Could you check a few things on this drawing? It's one solid part, dimensions in mm from its lowest x, y, z. A direction names the side the tool comes from. Give positions to 0.01 mm unless a question says otherwise; leave off trailing zeros. Write each loop counter-clockwise with the first axis right and the second up, starting at its lowest first coordinate (ties: lowest second). Pieces come first, ordered by that corner, then holes. Notation, with made-up numbers: M 88.25,24.5 L 109.25,24.5 A17 ccw 109.25,44.5 Z; hole C 32.25,16 d2. An arc over 180 degrees is marked long. Write each question's results on one line, items separated by ' | '.
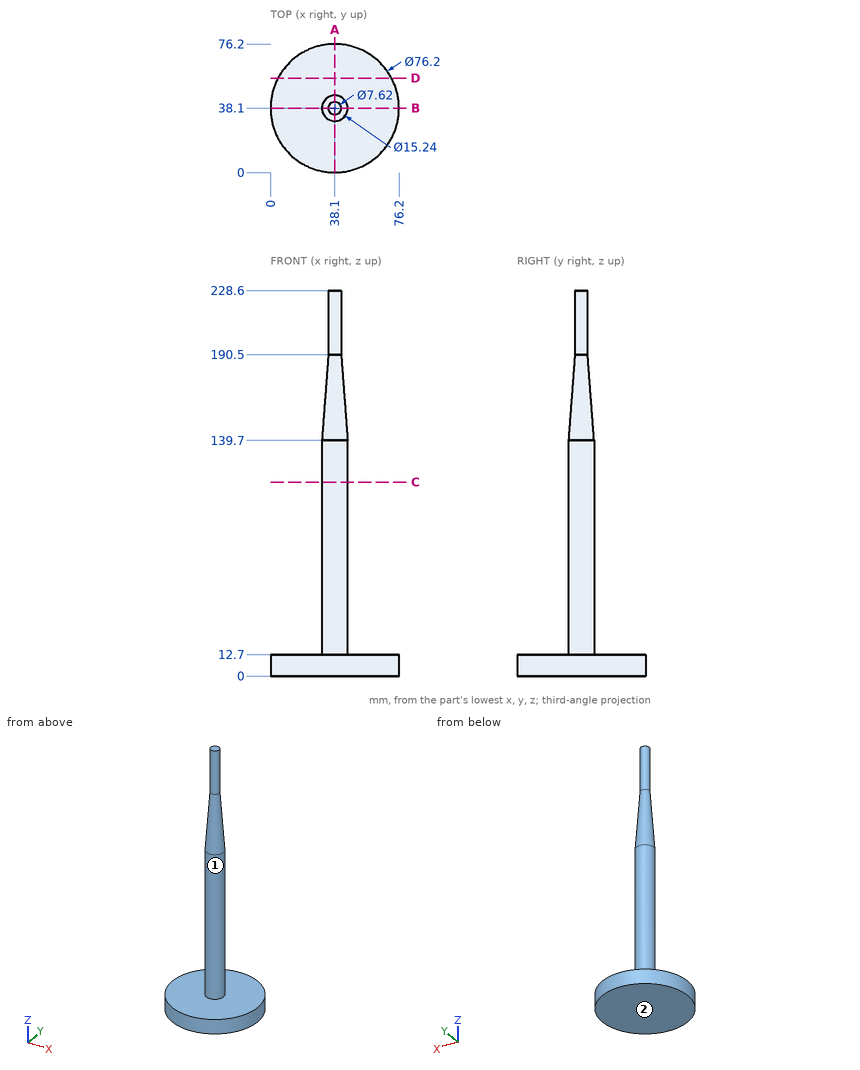
Item 1: For the marked faces 1 and 2, which set-ups out of +Z, -Z, +X, -X, +Y, -Y let a thin tool reach every point of the face, with its end or its side?
Geometry says:
face 1: +Z | face 2: -Z, +X, -X, +Y, -Y
Item 2: I want a section at D-D, the plane y = 56. Please give me the cut outline in (x, z).
Geometry says:
outline: M 4.47,0 L 71.73,0 L 71.73,12.7 L 4.47,12.7 Z
Item 3: I'm going to push flat-ended pins straight in: pin 1 (4 mm diameter, centred on x = 29.5, z = 75, fed in from +Y); pin 2 (10 mm diameter, centred on y = 35, z = 177.5, fed in from +X); pin 3 (10 mm diameter, centred on y = 46.5, z = 69, fed in from +X). Where does each tip first touch, or does it pass through?
Geometry says:
pin 1: stops at y = 41.91 | pin 2: stops at x = 43.19 | pin 3: stops at x = 44.92
Item 4: If I drill on line 1 (Z direction, x = 24, y = 31); line 2 (Y direction, x = 37, z = 87); line 3 (X direction, y = 43, z = 90), over which ranges is the centre line in solid material (lowest first)? Write a range as from..to.
Geometry says:
line 1: z = 0..12.7 | line 2: y = 30.56..45.64 | line 3: x = 32.26..43.94
Item 5: I want a section at A-A, the plane x = 38.1. Please give me the cut outline in (y, z).
Geometry says:
outline: M 0,0 L 76.2,0 L 76.2,12.7 L 45.72,12.7 L 45.72,139.7 L 41.91,190.5 L 41.91,228.6 L 34.29,228.6 L 34.29,190.5 L 30.48,139.7 L 30.48,12.7 L 0,12.7 Z
Item 6: I want a section at C-C, the plane z = 115. Please give me the cut outline in (x, y), and give its area (3 significant figures).
Geometry says:
outline: C 38.1,38.1 d15.24 | area: 182 mm2
